For this review, take the finished solid that the model builds, in its own axes (mm). A direction names the side the tool comes from. Coordinates: 2 decimals unless noted, no trailing zeros. Order: outer loops, then holes, each group sorted by start corner. A loop starts at its lowest first (then second) coordinate and runs counter-clockwise, first axis right, second up. Notation, with made-up numbers: (10, -22.75) -> (47, -22.75) arc R13 ccw to (47, -8.75) -> close; hole circle Ø3 at (-19.5, 67). An arc over 180 degrees is marked (long way). Return JSON: item names as keys, results as strings. Group by question number.
Item 1: Machinability: for faces 1 (the flat face through (-76.2, -50, 67)), 2 (the flat face through (95, -50, 12.7)), 3 (the flat face through (-31.75, -77, 52)), which of the approach directions +Z, -Z, +X, -X, +Y, -Y give a long, thin tool a straight path to every point of the face, cutting with its end or side? Answer none if there is none.
Item 2: Take a section at B-B (z = 59.5). Write out the cut boundary in (x, y).
Item 3: Take a section at A-A (y = -93.5). Write out the cut boundary in (x, z).
Item 4: Insertion check: pin 1 (12 mm diameter, centred on y = -27.5, z = 29.5, fed in from +X); pin 2 (10 mm diameter, centred on x = 95.5, y = -68.5, fed in from +Z); pin 3 (6 mm diameter, centred on x = -29, z = 54, fed in from +Y); pin 4 (8 mm diameter, centred on x = -4.5, z = 30.5, fed in from -Y). Each pin has a flat end and moves straight along its axis. Give the tip position at first contact, or say it passes through.
Item 5: Take a section at D-D (y = -46). Write out the cut boundary in (x, z).
Item 6: Take a section at C-C (x = -85). Write out the cut boundary in (y, z).
Item 7: For line 1 along X through (y, z) = (-17.5, 28.5); line 2 along Y through (x, z) = (74, 17); line 3 along Y through (x, z) = (15.5, 44.5), list the stretches that pass through material, from the lowest coordinate up.
```python
from build123d import *

# Parameters (mm, degrees)
F1_DEPTH = 101.6
F3_DEPTH = 120.65


with BuildPart() as f1:
    # F0 (on Front) → F1 (new body)
    with BuildSketch(Plane.XZ):
        Polygon((-101.6, 0), (0, 0), (101.6, 0), (101.6, 12.7), (88.9, 12.7), (88.9, 76.2), (-76.2, 76.2), (-76.2, 57.15), (-101.6, 57.15), align=None)
    extrude(amount=F1_DEPTH)

    # F2 (on face) → F3 (cut)
    with BuildSketch(Plane.YZ.offset(88.9)):
        Polygon((-101.6, 76.2), (-101.6, 12.7), (-38.1, 76.2), align=None)
    extrude(amount=-F3_DEPTH, mode=Mode.SUBTRACT)


solid = f1.part
```
Findings below:
{
 "1": {"face 1": "+Z, -X, +Y, -Y", "face 2": "+Z, +X, +Y, -Y", "face 3": "+Z, +X, -Y"},
 "2": {"outline": "(-76.2, -101.6) -> (-31.75, -101.6) -> (-31.75, -54.8) -> (88.9, -54.8) -> (88.9, 0) -> (-76.2, 0) -> close"},
 "3": {"outline": "(-101.6, 0) -> (101.6, 0) -> (101.6, 12.7) -> (88.9, 12.7) -> (88.9, 20.8) -> (-31.75, 20.8) -> (-31.75, 76.2) -> (-76.2, 76.2) -> (-76.2, 57.15) -> (-101.6, 57.15) -> close"},
 "4": {"pin 1": "stops at x = 88.9", "pin 2": "stops at z = 12.7", "pin 3": "stops at y = 0", "pin 4": "stops at y = -87.8"},
 "5": {"outline": "(-101.6, 0) -> (101.6, 0) -> (101.6, 12.7) -> (88.9, 12.7) -> (88.9, 68.3) -> (-31.75, 68.3) -> (-31.75, 76.2) -> (-76.2, 76.2) -> (-76.2, 57.15) -> (-101.6, 57.15) -> close"},
 "6": {"outline": "(-101.6, 0) -> (0, 0) -> (0, 57.15) -> (-101.6, 57.15) -> close"},
 "7": {"line 1": "x = -101.6 to 88.9", "line 2": "y = -97.3 to 0", "line 3": "y = -69.8 to 0"}
}
